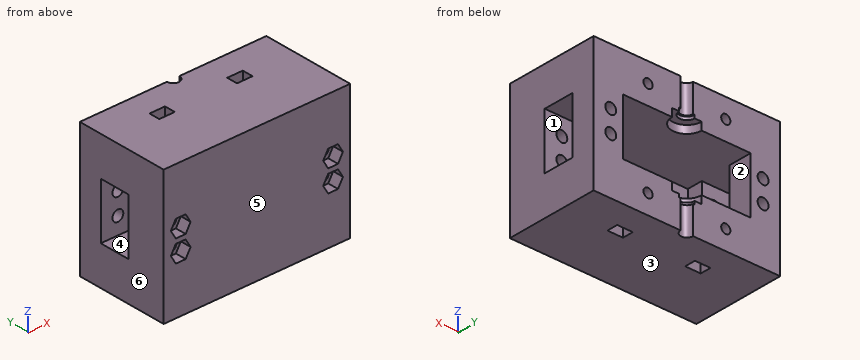
Autodesk Inventor part; units mm, degrees
ref_plane "YZ Plane" through (0, 0, 0) normal (1, 0, 0) x (0, 1, 0)
ref_plane "XZ Plane" through (0, 0, 0) normal (0, 1, 0) x (-1, 0, 0)
ref_plane "XY Plane" through (0, 0, 0) normal (0, 0, 1) x (1, 0, 0)
sketch "Schizzo1" plane through (0, 0, 0) normal (0, 1, 0) x (-1, 0, 0)
  line L0 (60, 43) -> (-60, 43)
  line L1 (-60, 43) -> (-60, -43)
  line L2 (-60, -43) -> (60, -43)
  line L3 (60, -43) -> (60, 43)
  line L4 (60, 43) -> (-60, -43) construction
  line L5 (-60, 43) -> (60, -43) construction
  point P0 (0, 0)
  point P1 (0, 0)
  point P2 (0, 0)
  dimension "d0" = 120
  dimension "d1" = 86
extrude "Estrusione1" add sketch "Schizzo1" along normal blind 60
sketch "Schizzo2" plane through (60, 0, 43) normal (1, 0, 0) x (0, 0, -1)
  line L0 (43, 0) -> (43, 15)
  line L1 (25, 45) -> (61, 45)
  line L2 (61, 45) -> (61, 15)
  line L3 (61, 15) -> (25, 15)
  line L4 (25, 15) -> (25, 45)
  line L5 (25, 45) -> (61, 15) construction
  line L6 (61, 45) -> (25, 15) construction
  point P0 (43, 30)
  dimension "d4" = 15
  dimension "d5" = 36
  dimension "d6" = 30
extrude "Estrusione2" cut sketch "Schizzo2" against normal blind 120
sketch "Schizzo3" plane through (60, 15, -18) normal (0, 0, 1) x (1, 0, 0)
  circle A0 centre (-60, 45) radius 9.5
  line L0 (0, 45) -> (-120, 45)
  point P0 (-60, -15)
  dimension "d9" = 19
extrude "Estrusione3" cut sketch "Schizzo3" against normal blind 5
sketch "Schizzo4" plane through (60, 15, -23) normal (0, 0, 1) x (1, 0, 0)
  circle A0 centre (-60, 45) radius 4
  line L0 (0, 45) -> (-120, 45)
  point P0 (-60, -15)
  dimension "d12" = 8
extrude "Estrusione4" cut sketch "Schizzo4" against normal blind 20
sketch "Schizzo5" plane through (60, 15, 18) normal (0, 0, -1) x (-1, 0, 0)
  circle A0 centre (60, 45) radius 9.5
  line L0 (120, 45) -> (0, 45)
  point P0 (60, -15)
  dimension "d15" = 19
extrude "Estrusione5" cut sketch "Schizzo5" against normal blind 5
sketch "Schizzo6" plane through (60, 15, 23) normal (0, 0, -1) x (-1, 0, 0)
  circle A0 centre (60, 45) radius 4
  line L0 (50.5, 45) -> (69.5, 45)
  point P0 (60, -15)
extrude "Estrusione6" cut sketch "Schizzo6" against normal blind 20
sketch "Schizzo7" plane through (0, 60, 0) normal (0, 1, 0) x (1, 0, 0)
  line L0 (-4, 43) -> (4, 43)
  line L1 (0, 43) -> (0, 18)
  line L2 (60, 18) -> (-60, 18)
  line L3 (0, -18) -> (0, -43)
  line L4 (4, -43) -> (-4, -43)
  line L5 (-133, 18) -> (-97, 18) construction
  line L6 (-25, 30.5) -> (25, 30.5)
  line L7 (-25, -30.5) -> (25, -30.5)
  point P0 (0, 0)
  point P1 (0, 30.5)
  point P2 (0, -30.5)
  point P3 (-50, 18)
  dimension "d22" = 50
  dimension "d23" = 50
hole "Foro1" at (-25, 60, -30.5) at (-25, 60, 30.5) at (25, 60, 30.5) at (25, 60, -30.5) direction (0, -1, 0) diameter 5.9 depth 35 tip angle 118
sketch "Schizzo8" plane through (-60, 0, 43) normal (0, 0, 1) x (1, 0, 0)
  line L0 (32.05, 60) -> (37.95, 60)
  line L1 (82.05, 60) -> (87.95, 60)
  line L2 (85, 60) -> (85, 40)
  line L3 (85, 60) -> (65, 60) construction
  line L4 (35, 60) -> (35, 40)
  line L5 (35, 60) -> (15, 60) construction
  line L6 (30, 43.5) -> (40, 43.5)
  line L7 (40, 43.5) -> (40, 36.5)
  line L8 (40, 36.5) -> (30, 36.5)
  line L9 (30, 36.5) -> (30, 43.5)
  line L10 (30, 43.5) -> (40, 36.5) construction
  line L11 (40, 43.5) -> (30, 36.5) construction
  line L12 (80, 43.5) -> (90, 43.5)
  line L13 (90, 43.5) -> (90, 36.5)
  line L14 (90, 36.5) -> (80, 36.5)
  line L15 (80, 36.5) -> (80, 43.5)
  line L16 (80, 43.5) -> (90, 36.5) construction
  line L17 (90, 43.5) -> (80, 36.5) construction
  point P0 (60, 0)
  point P1 (35, 40)
  dimension "d31" = 90
  dimension "d32" = 270
  dimension "d33" = 20
  dimension "d34" = 20
  dimension "d35" = 7
  dimension "d36" = 7
  dimension "d37" = 10
  dimension "d38" = 10
extrude "Estrusione7" cut sketch "Schizzo8" against normal blind 19
sketch "Schizzo10" plane through (60, 0, -43) normal (0, 0, -1) x (-1, 0, 0)
  line L0 (85, 60) -> (85, 40)
  line L1 (85, 60) -> (65, 60) construction
  line L2 (35, 60) -> (35, 40)
  line L3 (35, 60) -> (15, 60) construction
  line L4 (30, 43.5) -> (40, 43.5)
  line L5 (40, 43.5) -> (40, 36.5)
  line L6 (40, 36.5) -> (30, 36.5)
  line L7 (30, 36.5) -> (30, 43.5)
  line L8 (30, 43.5) -> (40, 36.5) construction
  line L9 (40, 43.5) -> (30, 36.5) construction
  line L10 (80, 43.5) -> (90, 43.5)
  line L11 (90, 43.5) -> (90, 36.5)
  line L12 (90, 36.5) -> (80, 36.5)
  line L13 (80, 36.5) -> (80, 43.5)
  line L14 (80, 43.5) -> (90, 36.5) construction
  line L15 (90, 43.5) -> (80, 36.5) construction
  line L16 (32.05, 60) -> (37.95, 60)
  line L17 (82.05, 60) -> (87.95, 60)
  point P0 (60, 0)
  point P1 (50, 0)
  point P2 (35, 40)
  dimension "d42" = 90
  dimension "d43" = 270
  dimension "d44" = 20
  dimension "d45" = 20
  dimension "d46" = 7
  dimension "d47" = 7
  dimension "d48" = 10
  dimension "d49" = 10
extrude "Estrusione8" cut sketch "Schizzo10" against normal blind 19
sketch "Schizzo11" plane through (60, 15, 18) normal (0, 0, -1) x (-1, 0, 0)
  line L0 (30.0078, 67.5) -> (89.9922, 22.5) construction
  line L1 (90.0057, 68) -> (30.1859, 18.1994) construction
  line L2 (56, 45) -> (0, 45)
  line L3 (120, 45) -> (64, 45)
  line L4 (0, 45) -> (120, 45)
  line L5 (60, 45) -> (290, 45) construction
  line L6 (60, 45) -> (60, 19)
  line L7 (60, 45) -> (86, 45) construction
  line L8 (60, 19) -> (92.5948, 19) construction
  line L9 (60, 19) -> (90, 19)
  line L10 (60, 19) -> (90, 19) construction
  line L11 (60, 19) -> (30, 19)
  line L12 (32.05, 10) -> (32.05, 21.5)
  line L13 (60, 19) -> (90, 19) construction
  line L14 (60, 45) -> (60, 68)
  line L15 (60, 68) -> (90.0057, 68)
  line L16 (90.0057, 68) -> (30, 68)
  line L17 (30, 68) -> (30, 19)
  line L18 (30, 19) -> (90.0057, 19)
  line L19 (90.0057, 19) -> (90.0057, 68)
  circle A0 centre (60, 45) radius 39.7032
  point P0 (60, -15)
  point P1 (61.2511, 44.0615)
  dimension "d52" = 60
  dimension "d53" = 45.5
  dimension "d72" = 26
  dimension "d73" = 90
  dimension "d75" = 30
  dimension "d76" = 0
  dimension "d77" = 30
  dimension "d78" = 180
  dimension "d79" = 23
sketch "Schizzo12" plane through (60, 15, 18) normal (0, 0, -1) x (-1, 0, 0)
  line L0 (120, -15) -> (120, 45)
  line L1 (120, 45) -> (120, 32)
  line L2 (120, 45) -> (133, 45) construction
  line L3 (120, 32) -> (150, 32)
  line L4 (150, 32) -> (150, 35)
  line L5 (61.2511, 44.0615) -> (261.2511, 44.0615) construction
  arc A0 (56, 45) -> (64, 45) centre (60, 45) ccw
  line L6 (60, 45) -> (233.2051, 145)
  line L7 (60, 45) -> (260, 45) construction
  line L8 (150, 35) -> (350, 35) construction
  line L9 (155, 82.5278) -> (145, 99.8483)
  line L10 (150, 35) -> (206.188, 35) construction
  line L11 (155, 82.5278) -> (138, 72.7128)
  line L12 (150, 32) -> (150, 79.641)
  line L13 (150, 79.641) -> (150, 32)
  circle A1 centre (150, 76.1769) radius 3
  line L14 (150, 32) -> (150, 76.1769)
  line L15 (150, 32) -> (120, 10)
  line L16 (60, 45) -> (60, 245)
  line L17 (69.5, 45) -> (50.5, 45)
  line L18 (60, 45) -> (260, 45) construction
  arc A2 (77.4356, 61) -> (42.5644, 61) centre (60, 46) ccw
  circle A3 centre (60, 46) radius 23
  line L19 (60, 45) -> (-140, 45)
  line L20 (60, 45) -> (260, 45) construction
  line L21 (120, 45) -> (64, 45)
  circle A4 centre (233.2051, 145) radius 151.0476
  point P0 (60, -15)
  point P1 (61.2511, 44.0615)
  point P2 (61.2511, 44.0615)
  point P3 (60, 69)
  point P4 (0, 45)
  point P5 (102.394, 69.4762)
  dimension "d54" = 13
  dimension "d55" = 90
  dimension "d56" = 30
  dimension "d57" = 90
  dimension "d58" = 3
  dimension "d61" = 200
  dimension "d62" = 30
  dimension "d66" = 20
  dimension "d67" = 47.641
  dimension "d68" = 6
  dimension "d69" = 44.1769
  dimension "d173" = 200
  dimension "d174" = 90
  dimension "d175" = 176
  dimension "d176" = 200
  dimension "d177" = 180
  dimension "d178" = 140
  dimension "d179" = 302.0953
sketch "Schizzo13" plane through (0, 60, 0) normal (0, 1, 0) x (1, 0, 0)
  line L0 (-41, -18) -> (41, -18)
  line L1 (41, -18) -> (41, 18)
  line L2 (41, 18) -> (-41, 18)
  line L3 (-41, 18) -> (-41, -18)
  line L4 (-41, -18) -> (41, 18) construction
  line L5 (41, -18) -> (-41, 18) construction
  point P0 (0, 0)
  point P1 (0, 0)
  point P2 (0, 0)
  dimension "d132" = 82
  dimension "d133" = 36
extrude "Estrusione9" cut sketch "Schizzo13" against normal blind 20
sketch "Schizzo16" plane through (60, 15, -23) normal (0, 0, 1) x (1, 0, 0)
  circle A0 centre (-60, 45) radius 5
  arc A1 (-64, 45) -> (-56, 45) centre (-60, 45) ccw
  point P0 (-60, -15)
  dimension "d94" = 10
extrude "Estrusione11" cut sketch "Schizzo16" against normal blind 2
sketch "Schizzo17" plane through (60, 15, 23) normal (0, 0, -1) x (-1, 0, 0)
  arc A0 (56, 45) -> (64, 45) centre (60, 45) ccw
  circle A1 centre (60, 45) radius 5
  point P0 (60, -15)
  dimension "d97" = 10
extrude "Estrusione12" cut sketch "Schizzo17" against normal blind 2
sketch "Schizzo21" plane through (60, 15, 18) normal (0, 1, 0) x (1, 0, 0)
  line L0 (-19, 36) -> (-19, 0)
  line L1 (-101, 0) -> (-101, 36)
  line L2 (-19, 0) -> (-50.5, 0)
  line L3 (-50.5, 36) -> (-19, 36)
  line L4 (-101, 36) -> (-69.5, 36)
  line L5 (-69.5, 0) -> (-101, 0)
  line L6 (-19, 36) -> (-19, 0)
  line L7 (-19, 0) -> (0, 0)
  line L8 (0, 0) -> (0, 36)
  line L9 (0, 36) -> (-19, 36)
  line L10 (-101, 36) -> (-101, 0)
  line L11 (-101, 0) -> (-120, 0)
  line L12 (-120, 0) -> (-120, 36)
  line L13 (-120, 36) -> (-101, 36)
  line L14 (-120, 61) -> (-120, -25)
  line L15 (0, -25) -> (0, 61)
  point P0 (-60, 18)
extrude "Estrusione14" add sketch "Schizzo21" along normal blind 10
sketch "Schizzo15" plane through (0, 60, 0) normal (0, 1, 0) x (1, 0, 0)
  line L0 (-60, 43) -> (-60, -43)
  line L1 (60, -43) -> (60, 43)
  line L2 (60, 0) -> (66, 0) construction
  line L3 (-60, -18) -> (-60, 18)
  line L4 (-49, 0) -> (-42, 0) construction
  line L5 (-49, 0) -> (-42, 0) construction
  line L6 (-43, 0) -> (-49, 0)
  line L7 (43, 0) -> (49, 0)
  line L8 (43, 0) -> (49, 0) construction
  line L9 (-49, 0) -> (-49, 7)
  line L10 (-49, 0) -> (-42, 0) construction
  line L11 (-49, 0) -> (-49, -7)
  line L12 (-49, 0) -> (-42, 0) construction
  line L13 (49, 0) -> (49, 7)
  line L14 (49, 0) -> (56, 0) construction
  line L15 (49, 0) -> (49, -7)
  line L16 (49, 0) -> (56, 0) construction
  point P0 (0, 0)
  dimension "d134" = 6
  dimension "d137" = 6
  dimension "d138" = 0
  dimension "d139" = 7
  dimension "d140" = 90
  dimension "d141" = 7
  dimension "d142" = 90
  dimension "d143" = 7
  dimension "d144" = 90
  dimension "d145" = 7
  dimension "d146" = 90
hole "Foro5" at (49, 60, 7) at (49, 60, -7) at (-49, 60, 7) at (-49, 60, -7) direction (0, -1, 0) diameter 7 depth 60
sketch "Schizzo22" plane through (0, 0, 0) normal (0, -1, 0) x (1, 0, 0)
  circle A0 centre (-49, -7) radius 3.5
  circle A1 centre (-49, 7) radius 3.5
  circle A2 centre (49, -7) radius 3.5
  circle A3 centre (49, 7) radius 3.5
  circle A4 centre (-49, -7) radius 5.5
  circle A5 centre (-49, 7) radius 5.5
  circle A6 centre (49, -7) radius 5.5
  circle A7 centre (49, 7) radius 5.5
  line L0 (52.1754, -1.5) -> (55.3509, -7)
  line L1 (55.3509, -7) -> (52.1754, -12.5)
  line L2 (52.1754, -12.5) -> (45.8246, -12.5)
  line L3 (45.8246, -12.5) -> (42.6491, -7)
  line L4 (42.6491, -7) -> (45.8246, -1.5)
  line L5 (45.8246, -1.5) -> (52.1754, -1.5)
  line L6 (45.8246, 1.5) -> (42.6491, 7)
  line L7 (42.6491, 7) -> (45.8246, 12.5)
  line L8 (45.8246, 12.5) -> (52.1754, 12.5)
  line L9 (52.1754, 12.5) -> (55.3509, 7)
  line L10 (55.3509, 7) -> (52.1754, 1.5)
  line L11 (52.1754, 1.5) -> (45.8246, 1.5)
  line L12 (-45.8246, -1.5) -> (-42.6491, -7)
  line L13 (-42.6491, -7) -> (-45.8246, -12.5)
  line L14 (-45.8246, -12.5) -> (-52.1754, -12.5)
  line L15 (-52.1754, -12.5) -> (-55.3509, -7)
  line L16 (-55.3509, -7) -> (-52.1754, -1.5)
  line L17 (-52.1754, -1.5) -> (-45.8246, -1.5)
  line L18 (-52.1754, 1.5) -> (-55.3509, 7)
  line L19 (-55.3509, 7) -> (-52.1754, 12.5)
  line L20 (-52.1754, 12.5) -> (-45.8246, 12.5)
  line L21 (-45.8246, 12.5) -> (-42.6491, 7)
  line L22 (-42.6491, 7) -> (-45.8246, 1.5)
  line L23 (-45.8246, 1.5) -> (-52.1754, 1.5)
  point P0 (0, 0)
  point P1 (49, -1.5)
  point P2 (49, 1.5)
  point P3 (-49, -1.5)
  point P4 (-49, 1.5)
  dimension "d167" = 11
  dimension "d168" = 11
  dimension "d169" = 11
  dimension "d170" = 11
extrude "Estrusione15" cut sketch "Schizzo22" against normal blind 7 contours A0 | A1 | A2 | A3 | A4 | A4 L12 L13 | A4 L17 L12 | L13 L14 A4 | A4 L16 L17 | L14 L15 A4 | A4 L15 L16 | A5 | A5 L21 L22 | A5 L20 L21 | L22 L23 A5 | A5 L19 L20 | L23 L18 A5 | A5 L18 L19 | A6 | A6 L0 L1 | A6 L5 L0 | L1 L2 A6 | A6 L4 L5 | L2 L3 A6 | A6 L3 L4 | A7 | A7 L9 L10 | A7 L8 L9 | L10 L11 A7 | A7 L7 L8 | L11 L6 A7 | A7 L6 L7
properties part number "19_Base_Pezzo_Unico" material "PLA(Stampato)(D0,646)"
The model under review builds one solid part; all positions refer to its coordinate system, in mm. Face numbers are marked on the shaded views. A direction names the side the tool comes from. Round coordinates to 2 decimals unless told otherwise and drop trailing zeros. Order: outer loops, then holes, each group sorted by start corner. A loop starts at its lowest first (then second) coordinate and runs counter-clockwise, first axis right, second up.
(1) Tool access review of the marked faces 1, 2 and 3: name each direction out of +Z, -Z, +X, -X, +Y, -Y from which nothing blocks a thin tool from reaching the whole face with its end or side.
Working result:
face 1: +X, -X
face 2: +Y
face 3: -Z, +X, -X, +Y, -Y
(2) Take a section at B-B, the plane x = -49. Count the separate pieces of the cut face and the enclosed holes in it, plus the area to 3 significant figures.
Working result:
separate pieces: 4
enclosed holes: 0
area: 3,820 mm2
(3) Take a section at D-D, the plane z = -36.5. State the section outline as (x, y) points.
Working result:
outline: (-60, 0) - (60, 0) - (60, 60) - (4, 60) arc R4 cw to (-4, 60) - (-60, 60) - close; hole (-30, 36.5) - (-20, 36.5) - (-20, 43.5) - (-30, 43.5) - close; hole (20, 36.5) - (30, 36.5) - (30, 43.5) - (20, 43.5) - close
(4) For P1, Ø3.5, axis at x = -23, y = 39.5, coming from the -Z side; P2, Ø2, axis at x = 12, z = 11.5, coming from the +Y side; P3, Ø9, axis at x = -49, z = -7, coming from the -Y side; P4, Ø6.5, axis at x = 49, z = 7, coming from the +Y side, all flat-tipped, find the tip position at first contact; note any pin that passes through.
Working result:
P1: stops at z = -24
P2: stops at y = 15
P3: stops at y = 7
P4: passes through
(5) Take a section at A-A, the plane z = -15. State the section outline as (x, y) points.
Working result:
outline: (-60, 0) - (60, 0) - (60, 25) - (41, 25) - (41, 15) - (-41, 15) - (-41, 25) - (-60, 25) - close; (-60, 45) - (-41, 45) - (-41, 60) - (-60, 60) - close; (41, 45) - (60, 45) - (60, 60) - (41, 60) - close
(6) Mouldability with a two-part tool opening along X and no side actions: class the marked faces 4, 5 and 6 as released by +X, released by -X, zero draft, split by the parting line, or undercut.
Working result:
face 4: undercut
face 5: zero draft
face 6: released by -X
(7) Wall thickness on L1, parallel to Z at x = 25, y = 47.75; L2, parallel to X at y = 56, z = 7; L3, parallel to Z at x = 49, y = 49.75: over which ranges is each line inside the solid? List them lowest first.
Working result:
L1: z = -43 to -33.45, -27.55 to -18, 18 to 27.55, 33.45 to 43
L2: x = -60 to -52.5, -45.5 to -41, 41 to 45.5, 52.5 to 60
L3: z = -43 to -10.5, -3.5 to 3.5, 10.5 to 43
(8) Take a section at C-C, the plane y = 40. State the section outline as (x, z) points, plus the area to 3 significant figures.
Working result:
outline: (-60, -43) - (-30, -43) - (-30, -24) - (-20, -24) - (-20, -43) - (20, -43) - (20, -24) - (30, -24) - (30, -43) - (60, -43) - (60, -18) - (-60, -18) - close; (-60, 18) - (60, 18) - (60, 43) - (30, 43) - (30, 24) - (20, 24) - (20, 43) - (-20, 43) - (-20, 24) - (-30, 24) - (-30, 43) - (-60, 43) - close
area: 5,240 mm2
